Here's how the part is built. I have some questions about the finished solid (model axes, mm). Face numbers are marked on the shaded views. Round coordinates to 2 decimals unless told otherwise and drop trailing zeros. Order: outer loops, then holes, each group sorted by start corner. A loop starts at its lowest first (then second) coordinate and runs counter-clockwise, first axis right, second up. Notation, with made-up numbers: (26.25, 71) -> (81.25, 71) arc R27 cw to (81.25, 94) -> close; hole circle Ø1 at (77.25, 65). An arc over 180 degrees is marked (long way). Use a Markdown table: item, result. Add a question column.
(1) Thinking about a two-plate mould opening in Z: for the marked faces 1, 2 and 3, which applies, pulls with the +Z half, pulls with the -Z half, needs draft (parallel to the pull), parting line crosses it, or undercut?
(2) If I drill on probe 1 along Z at (x, y) = (0, -35.5); probe 2 along Z at (x, y) = (2, -27); probe 3 along X at (y, z) = (-9, 11), over which ranges is the centre line in solid material (lowest first)?
(3) I want a section at D-D, the plane x = 59. Please give me the cut outline in (y, z).
(4) I'm going to push flat-ended pins straight in: P1, Ø1, axis at x = 11.5, z = 12.5, coming from the -Y side; P2, Ø2, axis at y = -26.5, z = -16.5, coming from the -X side (3 decimals); P3, Ø1, axis at x = -46.5, z = -6, coming from the +Y side. Where does each tip first touch, or does it pass through?
(5) I want a section at C-C, the plane y = -23.5. Please give me the cut outline in (x, z).
(6) I want a section at A-A, the plane x = 0. Please give me the cut outline in (y, z).
(7) I want a section at B-B, the plane z = 0. Please give me the cut outline in (x, y).
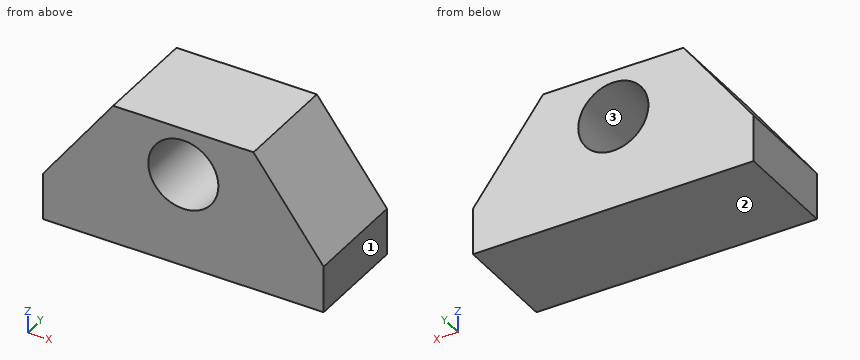
from build123d import *

# Parameters (mm, degrees)
F0_R     = 19.05
F1_DEPTH = 57.15


with BuildPart() as f1:
    # F0 (on Front) → F1 (new body)
    with BuildSketch(Plane.XZ):
        Polygon((-76.2, -25.4), (-76.2, -50.8), (76.2, -50.8), (76.2, -25.4), (38.1, 25.4), (0, 25.4), (-38.1, 25.4), align=None)
        Circle(F0_R, mode=Mode.SUBTRACT)
    extrude(amount=F1_DEPTH)


solid = f1.part
Taken from the geometry:
| question | item | result |
|---|---|---|
| 1 | face 1 | needs draft |
| 1 | face 2 | pulls with the -Z half |
| 1 | face 3 | undercut |
| 2 | probe 1 | z = -50.8 to -19.05, 19.05 to 25.4 |
| 2 | probe 2 | z = -50.8 to -18.94, 18.94 to 25.4 |
| 2 | probe 3 | x = -48.9 to -15.55, 15.55 to 48.9 |
| 3 | outline | (-57.15, -50.8) -> (0, -50.8) -> (0, -2.47) -> (-57.15, -2.47) -> close |
| 4 | P1 | passes through |
| 4 | P2 | stops at x = -70.275 |
| 4 | P3 | stops at y = 0 |
| 5 | outline | (-76.2, -50.8) -> (76.2, -50.8) -> (76.2, -25.4) -> (38.1, 25.4) -> (-38.1, 25.4) -> (-76.2, -25.4) -> close; hole circle Ø38.1 at (0, 0) |
| 6 | outline | (-57.15, -50.8) -> (0, -50.8) -> (0, -19.05) -> (-57.15, -19.05) -> close; (-57.15, 19.05) -> (0, 19.05) -> (0, 25.4) -> (-57.15, 25.4) -> close |
| 7 | outline | (-57.15, -57.15) -> (-19.05, -57.15) -> (-19.05, 0) -> (-57.15, 0) -> close; (19.05, -57.15) -> (57.15, -57.15) -> (57.15, 0) -> (19.05, 0) -> close |
